Check sheet for the drawn part. Datum: minimum x, y, z corner. Units: mm. A direction names the side the tool comes from. Coordinates: 2 decimals unless noted, no trailing zeros. Write each loop counter-clockwise with the first axis right and the second up, starting at its lowest first coordinate (ties: lowest second). Pieces come first, ordered by that corner, then holes. Notation, with made-up numbers: (27, 4.25) -> (65, 4.25) arc R23 cw to (65, 37.25) -> close; hole circle Ø1 at (79, -26). An arc over 180 degrees is marked (long way). Answer in a Markdown table with one row per item. Add a question column.
1. Set-up check for the marked faces 4 and 5: record each of +Z, -Z, +X, -X, +Y, -Y from which the full face is reachable in a straight line by a thin tool's end or side.
2. Cross-section at D-D on y = 12.5. Record the cut outline in (x, z).
3. Cross-section at B-B on z = 0.8. Record the cut outline in (x, y).
4. Scan lines: L1, parallel to Y at x = 12.75, z = 0.45; L2, parallel to X at y = 11.5, z = 2.2; L3, parallel to Y at x = 7.5, z = 1.5. Record each from-to range of solid material in increasing order. Write a range as from..to.
5. Cross-section at A-A on y = 7.5. Record the cut outline in (x, z), and give its area (3 significant figures).
6. Mould release check, pull along Y, two halves, no side actions. Record for the marked faces 1, 2 and 3: pulls with the +Y half, pulls with the -Y half, needs draft (parallel to the pull), parting line crosses it, or undercut.
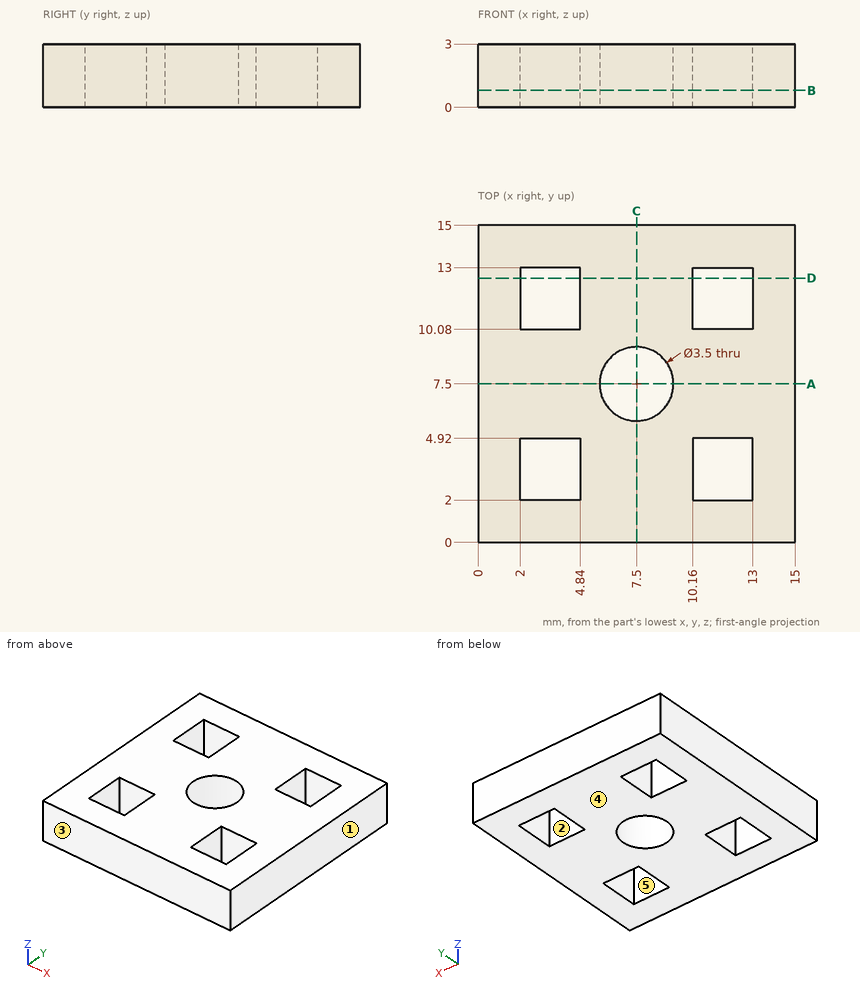
Results found:
| question | item | result |
|---|---|---|
| 1 | face 4 | -Z, +X, -X, +Y, -Y |
| 1 | face 5 | +Z, -Z |
| 2 | outline | (0, 0) -> (2, 0) -> (2, 3) -> (0, 3) -> close; (4.84, 0) -> (10.16, 0) -> (10.16, 3) -> (4.84, 3) -> close; (13, 0) -> (15, 0) -> (15, 3) -> (13, 3) -> close |
| 3 | outline | (0, 0) -> (15, 0) -> (15, 15) -> (0, 15) -> close; hole (2, 2) -> (4.84, 2) -> (4.84, 4.92) -> (2, 4.92) -> close; hole (2, 10.08) -> (4.84, 10.08) -> (4.84, 13) -> (2, 13) -> close; hole circle Ø3.5 at (7.5, 7.5); hole (10.16, 2) -> (13, 2) -> (13, 4.92) -> (10.16, 4.92) -> close; hole (10.16, 10.08) -> (13, 10.08) -> (13, 13) -> (10.16, 13) -> close |
| 4 | L1 | y = 0..2, 4.92..10.08, 13..15 |
| 4 | L2 | x = 0..2, 4.84..10.16, 13..15 |
| 4 | L3 | y = 0..5.75, 9.25..15 |
| 5 | outline | (0, 0) -> (5.75, 0) -> (5.75, 3) -> (0, 3) -> close; (9.25, 0) -> (15, 0) -> (15, 3) -> (9.25, 3) -> close |
| 5 | area | 34.5 mm^2 |
| 6 | face 1 | needs draft |
| 6 | face 2 | undercut |
| 6 | face 3 | pulls with the -Y half |
